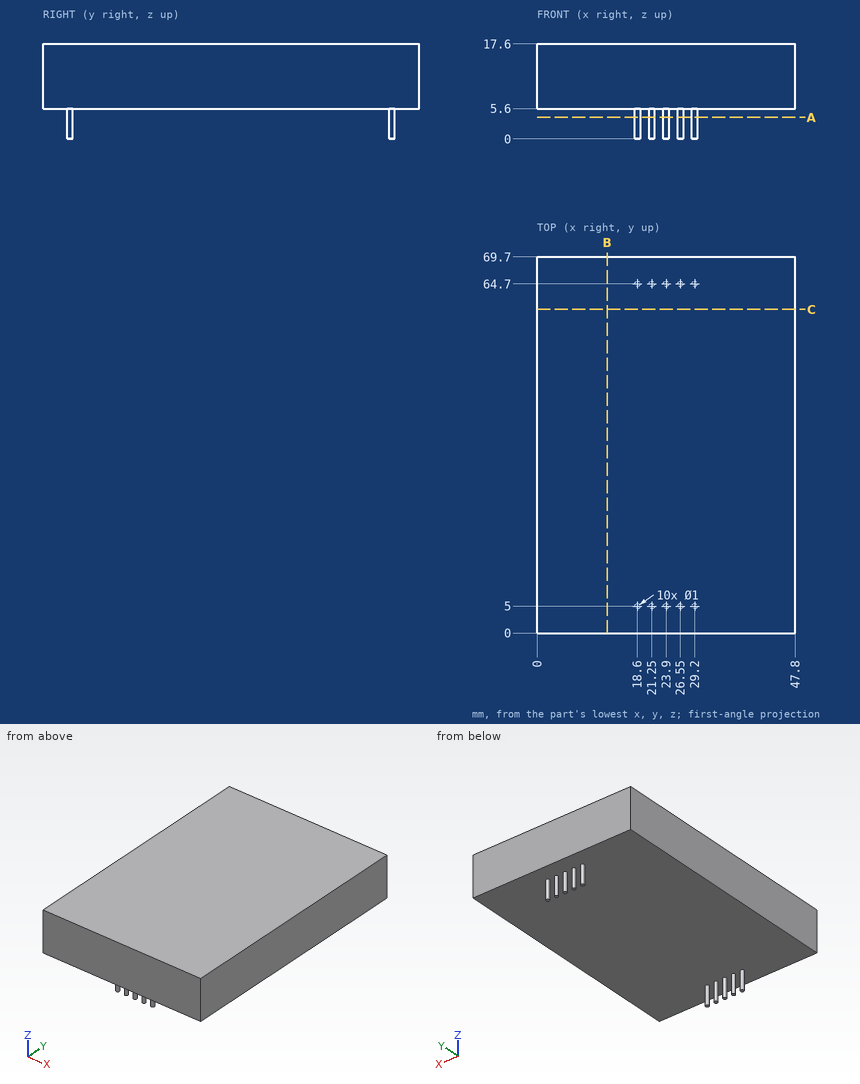
Can you work these out from the drawing? Everything is in mm from the part's minimum corner. Give positions to 0.01 mm unless a question says otherwise; leave off trailing zeros. Order: outer loops, then holes, each group sorted by start corner. A loop starts at its lowest first (then second) coordinate and runs counter-clockwise, first axis right, second up. Notation, with made-up numbers: M 54,38.5 L 67,38.5 A8 ccw 67,48.5 Z; hole C 84,-35 d2. An arc over 180 degrees is marked long. Use a Markdown table: item, result. Add a question column.
1. Suppose I cut it at C-C (y = 60). List the corners of the cut face in (x, z) for me.
2. For pin 1 Ø8 at (x, z) = (32, 12) entering from -Y; pin 2 Ø14.5 at (x, y) = (21, 26.5) entering from -Z, each with a flat end and sliding along its axis, tell me the tip position at first contact or that it passes through.
3. I need wall thicknesses on probe 1 along Z at (x, y) = (2, 12.5). Which ranges of the line are inside material? Lowest first, please. Write a range as from..to.
4. Suppose I cut it at B-B (x = 13). List the corners of the cut face in (y, z) for me.
5. Suppose I cut it at A-A (z = 4). Give the number of separate pieces and of enclosed holes in the cut face, and give its area (3 significant figures).
Results list:
| question | item | result |
|---|---|---|
| 1 | outline | M 0,5.6 L 47.8,5.6 L 47.8,17.6 L 0,17.6 Z |
| 2 | pin 1 | stops at y = 0 |
| 2 | pin 2 | stops at z = 5.6 |
| 3 | probe 1 | z = 5.6..17.6 |
| 4 | outline | M 0,5.6 L 69.7,5.6 L 69.7,17.6 L 0,17.6 Z |
| 5 | separate pieces | 10 |
| 5 | enclosed holes | 0 |
| 5 | area | 7.85 mm² |
